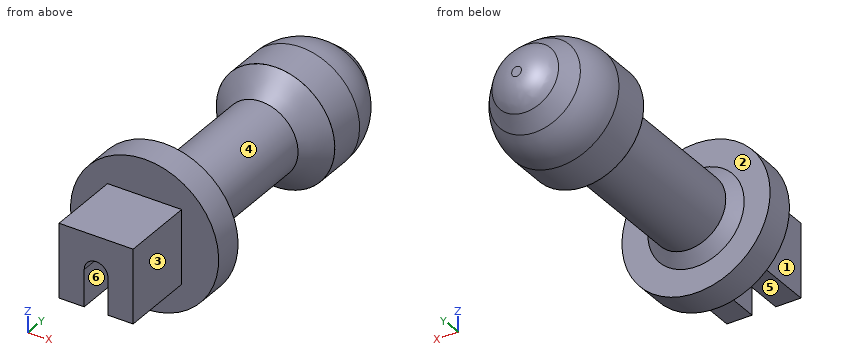
```python
from build123d import *

# Parameters (mm, degrees)
SKETCH1_W           = 10
SKETCH1_H           = 10
BOSS_EXTRUDE1_DEPTH = 10
SKETCH2_R           = 10
BOSS_EXTRUDE2_DEPTH = 4
SKETCH3_R           = 5
BOSS_EXTRUDE3_DEPTH = 23
CHAMFER1_SIZE       = 3
SKETCH7_R           = 1.6
CUT_EXTRUDE2_DEPTH  = 6
SKETCH8_W           = 6
SKETCH8_H           = 3
CUT_EXTRUDE3_DEPTH  = 8
CUT_EXTRUDE4_REACH  = 54.924
CHAMFER2_SIZE       = 1.5


with BuildPart() as part:
    # Sketch1 → Boss-Extrude1 (new body)
    with BuildSketch(Plane(origin=(0, 0, 0), x_dir=(1, 0, 0), z_dir=(0, 1, 0))):
        Rectangle(SKETCH1_W, SKETCH1_H)
    extrude(amount=BOSS_EXTRUDE1_DEPTH)

    # Sketch2 → Boss-Extrude2 (add)
    with BuildSketch(Plane(origin=(0, 10, 0), x_dir=(1, 0, 0), z_dir=(0, 1, 0))):
        with Locations(Location((0, 0, 0), (0, 0, 270))):
            Circle(SKETCH2_R)
    extrude(amount=BOSS_EXTRUDE2_DEPTH)

    # Sketch3 → Boss-Extrude3 (add)
    with BuildSketch(Plane(origin=(0, 14, 0), x_dir=(1, 0, 0), z_dir=(0, 1, 0))):
        with Locations(Location((0, 0, 0), (0, 0, 270))):
            Circle(SKETCH3_R)
    extrude(amount=BOSS_EXTRUDE3_DEPTH)

    # Sketch4 → Revolve1 (revolve)
    with BuildSketch(Plane.XY, mode=Mode.PRIVATE) as revolve1_sk:
        with BuildLine():
            Line((0, 37), (0, 51))
            Line((0, 51), (0.65812527, 51))
            ThreePointArc((0.65812527, 51), (2.778902251, 50.527947106), (4.499231668, 49.200921998))
            Line((4.499231668, 49.200921998), (6.145770237, 47.225075716))
            ThreePointArc((6.145770237, 47.225075716), (7.522172621, 44.827002629), (8, 42.103600519))
            Line((8, 42.103600519), (8, 37))
            Line((8, 37), (0, 37))
        make_face()
    revolve(revolve1_sk.sketch.rotate(Axis((0, 37, 0), (0, 1, 0)), 90), axis=Axis((0, 37, 0), (0, 1, 0)))

    # Chamfer1
    chamfer1_edges = [part.edges().sort_by_distance(p)[0] for p in [
        (0, 37, -5),
    ]]
    chamfer(chamfer1_edges, length=CHAMFER1_SIZE - 0.0001)  # a hair under: the kernel refuses the full size

    # Sketch7 → Cut-Extrude2 (cut)
    with BuildSketch(Plane.XZ):
        with Locations(Location((0, 0, 0), (0, 0, 270))):
            Circle(SKETCH7_R)
    extrude(amount=-CUT_EXTRUDE2_DEPTH, mode=Mode.SUBTRACT)

    # Sketch8 → Cut-Extrude3 (cut)
    with BuildSketch(Plane(origin=(0, 0, -5), x_dir=(-1, 0, 0), z_dir=(0, 0, -1))):
        with Locations((0, 7.5)):
            Rectangle(SKETCH8_W, SKETCH8_H)
    extrude(amount=-CUT_EXTRUDE3_DEPTH, mode=Mode.SUBTRACT)

    # Sketch9 → Cut-Extrude4 (cut, up to next)
    with BuildSketch(Plane.XZ, mode=Mode.PRIVATE) as cut_extrude4_sk1:
        with BuildLine():
            ThreePointArc((1.6, 0), (0, -1.6), (-1.6, 0))
            Line((-1.6, 0), (-1.6, -5))
            Line((-1.6, -5), (1.6, -5))
            Line((1.6, -5), (1.6, 0))
        make_face()
    cut_extrude4_tool1 = extrude(cut_extrude4_sk1.sketch, amount=-CUT_EXTRUDE4_REACH, mode=Mode.PRIVATE) & part.part
    add(cut_extrude4_tool1.solids().sort_by_distance((0, 0, -3.111284))[0], mode=Mode.SUBTRACT)

    # Chamfer2
    chamfer2_edges = [part.edges().sort_by_distance(p)[0] for p in [
        (0, 14, -5),
    ]]
    chamfer(chamfer2_edges, length=CHAMFER2_SIZE)


solid = part.part
```
Design review of the part built by this model. Coordinates are the model's own, in mm. Face numbers are marked on the shaded views. A direction names the side the tool comes from. Coordinates: 2 decimals unless noted, no trailing zeros. Write each loop counter-clockwise with the first axis right and the second up, starting at its lowest first coordinate (ties: lowest second). Pieces come first, ordered by that corner, then holes.
1) Add section A-A (y = 25). Write out the cut boundary in (x, z), plus the area to 3 significant figures.
2) Add section B-B (y = 43). Write out the cut boundary in (x, z), plus the area to 3 significant figures.
3) To check wall thickness, follow L1, parallel to Y at x = 8.75, z = 0; L2, parallel to Y at x = 3, z = 4.25; L3, parallel to X at y = 5, z = 0.75. State the ranges of each line that lie inside material, in increasing order.
4) Insertion check: pin 1 (5 mm diameter, centred on x = 0.5, y = 27, fed in from -Z); pin 2 (3.5 mm diameter, centred on y = 7.5, z = -1.5, fed in from +X); pin 3 (1.5 mm diameter, centred on x = 1, y = 7.5, fed in from -Z). Each pin has a flat end and moves straight along its axis. Give the tip position at first contact, or say it passes through.
5) Machinability: for the marked faces 1, 2 and 3, which of the approach directions +Z, -Z, +X, -X, +Y, -Y give a long, thin tool a straight path to every point of the face, cutting with its end or side? Answer none if there is none.
6) Mouldability with a two-part tool opening along X and no side actions: class the marked faces 4, 5 and 6 as +X half, -X half, draft (parallel to the pull), parting line (faces both ways), or undercut.
Check result:
1. outline: circle Ø10 at (0, 0)
1. area: 78.5 mm2
2. outline: circle Ø15.9 at (0, 0)
2. area: 199 mm2
3. L1: y = 10 to 14
3. L2: y = 0 to 15.3, 34.2 to 48.36
3. L3: x = -5 to -1.41, 1.41 to 5
4. pin 1: stops at z = -5
4. pin 2: stops at x = 5
4. pin 3: stops at z = 3
5. face 1: +Z, -Z, -X, -Y
5. face 2: none
5. face 3: +Z, -Z, +X, -Y
6. face 4: parting line
6. face 5: draft
6. face 6: undercut
